Verification items for the finished model (mm, model axes). A direction names the side the tool comes from. Coordinates: 2 decimals unless noted, no trailing zeros. Order: outer loops, then holes, each group sorted by start corner. A loop starts at its lowest first (then second) coordinate and runs counter-clockwise, first axis right, second up. Notation, with made-up numbers: (-12, -2.75) -> (17, -2.75) arc R4 ccw to (17, 4.25) -> close; hole circle Ø6 at (6, 60.25). An arc over 180 degrees is marked (long way). Write each question's results on one line, items separated by ' | '. Start each with the question number.
(1) Cross-section at C-C on y = 9.5. Enter the section's corners in (x, z), and give its area (3 significant figures).
(2) Cross-section at A-A on x = 0. Give the number of separate pieces and of enclosed holes in the cut face, and give its area (3 significant figures).
(3) Cross-section at B-B on z = 15.25. Enter the section's corners in (x, y).
(4) Go/stop test with flat-tipped pins: pin 1 (2.5 mm diameter, centred on y = -6, z = 5, fed in from +X); pin 2 (1.5 mm diameter, centred on y = 0.5, z = 15, fed in from +X); pin 3 (4 mm diameter, centred on y = -6.5, z = 15, fed in from -X). Record where each tip stops, or that it passes through.
(5) Draft check along Y on faces 1 (the flat face through (0, 7.312, 9)), 2 (the cylindrical face through (-7.289, 4.196, 4.056)), 3 (the cylindrical face through (-7.289, -8.196, 10.712)). Enter one of: +Y half, -Y half, draft (parallel to the pull), parting line (faces both ways), or undercut.
(6) Set-up check for faces 4 (the flat face through (-3.95, 5, 16)), 5 (the cylindrical face through (-3.649, -9.715, 15.965)), 6 (the flat face through (3.127, 12.678, 9.232)), 7 (the flat face through (0, -2.124, 1)), 8 (the cylindrical face through (7.289, 4.196, 4.056)): record each of +Z, -Z, +X, -X, +Y, -Y from which the full face is reachable in a straight line by a thin tool's end or side.
(7) Cross-section at D-D on z = 4. Enter the section's corners in (x, y).
(8) Thickness scan on probe 1 along Y at (x, z) = (0, 13); probe 2 along Y at (x, z) = (0.25, 13.5); probe 3 along Z at (x, y) = (0, -2.45). Record the ranges inside material, lowest first. Write a range as [from, to].
```python
from build123d import *

# Parameters (mm, degrees)
F0_W         = 18
F0_H         = 16
F0_W_2       = 7.2
F0_H_2       = 3.15
F1_DEPTH     = 8
F2_R         = 6
F4_R         = 2.1
F5_DEPTH     = 10
F7_R         = 2.15
F8_DEPTH     = 5.5
F9_DEPTH     = 2.5
F10_T1_DEPTH = 35.4995000042
F12_R        = 2.15
F13_DEPTH    = 5
F14_T1_DEPTH = 7.5071501803


# Not quite as in the source:
# - a fillet or chamfer that OpenCascade refuses, or shapes differently, is made with other operations: its cross-section is extruded or revolved along the edge and cut away or added


with BuildPart() as f1:
    # F0 (on Top) → F1 (new body)
    with BuildSketch(Plane.XY):
        with Locations((0, -2)):
            Rectangle(F0_W, F0_H)
        with Locations((0, -5.225)):
            Rectangle(F0_W_2, F0_H_2, mode=Mode.SUBTRACT)
        with BuildLine():
            ThreePointArc((-1.5, -2.1236760582), (-1.1958260743, 2.3086792761), (2.6, 0))
            ThreePointArc((2.6, 0), (2.3086792761, -1.1958260743), (1.5, -2.1236760582))
            ThreePointArc((1.5, -2.1236760582), (0, -2.6), (-1.5, -2.1236760582))
        make_face(mode=Mode.SUBTRACT)
        with BuildLine():
            Line((1.5, -2.1236760582), (-1.5, -2.1236760582))
            ThreePointArc((-1.5, -2.1236760582), (0, -2.6), (1.5, -2.1236760582))
        make_face()
    extrude(amount=F1_DEPTH)

    # F2
    f2_edges = [f1.edges().sort_by_distance(p)[0] for p in [
        (9, -10, 4),
        (-9, -10, 4),
        (9, 6, 4),
        (-9, 6, 4),
    ]]
    fillet(f2_edges, radius=F2_R)

    # F4 (on offset) → F5 (cut)
    with BuildSketch(Plane.XZ.offset(10)):
        with Locations((0, 4)):
            Circle(F4_R)
    extrude(amount=-F5_DEPTH, mode=Mode.SUBTRACT)

    # F7 (on offset) → F8 (join)
    with BuildSketch(Plane.XY.offset(8)):
        Polygon((-9, 20), (-9, 0), (-9, -4), (-9, -10), (-3, -10), (3, -10), (9, -10), (9, -4), (9, 0), (9, 20), align=None)
        with BuildLine():
            ThreePointArc((-1.5, -2.1236760582), (0, 2.6), (1.5, -2.1236760582))
            Line((1.5, -2.1236760582), (-1.5, -2.1236760582))
        make_face(mode=Mode.SUBTRACT)
        with BuildLine():
            ThreePointArc((2.075, 14.5), (3.5940054257, 12.9809945743), (4.15, 10.9059945743))
            ThreePointArc((4.15, 10.9059945743), (3.5940054257, 8.8309945743), (2.075, 7.3119891486))
            ThreePointArc((2.075, 7.3119891486), (0, 6.7559945743), (-2.075, 7.3119891486))
            ThreePointArc((-2.075, 7.3119891486), (-3.5940054257, 8.8309945743), (-4.15, 10.9059945743))
            ThreePointArc((-4.15, 10.9059945743), (-3.5940054257, 12.9809945743), (-2.075, 14.5))
            ThreePointArc((-2.075, 14.5), (0, 15.0559945743), (2.075, 14.5))
        make_face(mode=Mode.SUBTRACT)
        with BuildLine():
            ThreePointArc((-4.15, 10.9059945743), (-3.5940054257, 8.8309945743), (-2.075, 7.3119891486))
            Line((-2.075, 7.3119891486), (-4.15, 10.9059945743))
        make_face()
        with BuildLine():
            Line((-4.15, 10.9059945743), (-2.075, 14.5))
            ThreePointArc((-2.075, 14.5), (-3.5940054257, 12.9809945743), (-4.15, 10.9059945743))
        make_face()
        with BuildLine():
            Line((-2.075, 14.5), (2.075, 14.5))
            ThreePointArc((2.075, 14.5), (0, 15.0559945743), (-2.075, 14.5))
        make_face()
        with BuildLine():
            Line((2.075, 14.5), (4.15, 10.9059945743))
            ThreePointArc((4.15, 10.9059945743), (3.5940054257, 12.9809945743), (2.075, 14.5))
        make_face()
        with BuildLine():
            ThreePointArc((2.075, 7.3119891486), (3.5940054257, 8.8309945743), (4.15, 10.9059945743))
            Line((4.15, 10.9059945743), (2.075, 7.3119891486))
        make_face()
        with BuildLine():
            ThreePointArc((-2.075, 7.3119891486), (0, 6.7559945743), (2.075, 7.3119891486))
            Line((2.075, 7.3119891486), (-2.075, 7.3119891486))
        make_face()
        Polygon((2.075, 7.3119891486), (4.15, 10.9059945743), (2.075, 14.5), (-2.075, 14.5), (-4.15, 10.9059945743), (-2.075, 7.3119891486), align=None)
        with Locations((0, 10.9059945743)):
            Circle(F7_R, mode=Mode.SUBTRACT)
    extrude(amount=F8_DEPTH)

    # F7 (on offset) → F9 (cut)
    with BuildSketch(Plane.XY.offset(8)):
        Polygon((2.075, 7.3119891486), (4.15, 10.9059945743), (2.075, 14.5), (-2.075, 14.5), (-4.15, 10.9059945743), (-2.075, 7.3119891486), align=None)
        with Locations((0, 10.9059945743)):
            Circle(F7_R, mode=Mode.SUBTRACT)
    extrude(amount=F9_DEPTH, mode=Mode.SUBTRACT)

    # F10: fillet of radius 6 on 4 edges, made by hand

    # F10_s2 → F10_t1 (cut)
    with BuildSketch(Plane.XY.offset(-6.9997500021)):
        with BuildLine():
            ThreePointArc((-9.0001, -4.0001), (-7.2427406871, -8.2427406871), (-3.0001, -10.0001))
            Line((-3.0001, -10.0001), (-3.0001, -10.1201))
            ThreePointArc((-3.0001, -10.1201), (-6.00005, -10.12), (-9, -10.12))
            Line((-9, -10.12), (-9.12, -10))
            ThreePointArc((-9.12, -10), (-9.12, -7.00005), (-9.1201, -4.0001))
            Line((-9.1201, -4.0001), (-9.0001, -4.0001))
        make_face()
        with BuildLine():
            ThreePointArc((9.0001, -4.0001), (7.2427406871, -8.2427406871), (3.0001, -10.0001))
            Line((3.0001, -10.0001), (3.0001, -10.1201))
            ThreePointArc((3.0001, -10.1201), (6.00005, -10.12), (9, -10.12))
            Line((9, -10.12), (9.12, -10))
            ThreePointArc((9.12, -10), (9.12, -7.00005), (9.1201, -4.0001))
            Line((9.1201, -4.0001), (9.0001, -4.0001))
        make_face()
        with BuildLine():
            ThreePointArc((9.0001, 14.0001), (7.2427406871, 18.2427406871), (3.0001, 20.0001))
            Line((3.0001, 20.0001), (3.0001, 20.1201))
            ThreePointArc((3.0001, 20.1201), (6.00005, 20.12), (9, 20.12))
            Line((9, 20.12), (9.12, 20))
            ThreePointArc((9.12, 20), (9.12, 17.00005), (9.1201, 14.0001))
            Line((9.1201, 14.0001), (9.0001, 14.0001))
        make_face()
        with BuildLine():
            ThreePointArc((-9.0001, 14.0001), (-7.2427406871, 18.2427406871), (-3.0001, 20.0001))
            Line((-3.0001, 20.0001), (-3.0001, 20.1201))
            ThreePointArc((-3.0001, 20.1201), (-6.00005, 20.12), (-9, 20.12))
            Line((-9, 20.12), (-9.12, 20))
            ThreePointArc((-9.12, 20), (-9.12, 17.00005), (-9.1201, 14.0001))
            Line((-9.1201, 14.0001), (-9.0001, 14.0001))
        make_face()
    extrude(amount=F10_T1_DEPTH, mode=Mode.SUBTRACT)

    # F12 (on offset) → F13 (join)
    with BuildSketch(Plane.XY.offset(13.5)):
        with BuildLine():
            Line((-3.95, 19.9243143063), (-3.95, -9.9243143063))
            ThreePointArc((-3.95, -9.9243143063), (-3.4765050693, -9.9810486471), (-3, -10))
            Line((-3, -10), (3, -10))
            ThreePointArc((3, -10), (3.4765050693, -9.9810486471), (3.95, -9.9243143063))
            Line((3.95, -9.9243143063), (3.95, 19.9243143063))
            ThreePointArc((3.95, 19.9243143063), (3.4765050693, 19.9810486471), (3, 20))
            Line((3, 20), (-3, 20))
            ThreePointArc((-3, 20), (-3.4765050693, 19.9810486471), (-3.95, 19.9243143063))
        make_face()
        with BuildLine():
            Line((1.5, -2.1236760582), (-1.5, -2.1236760582))
            ThreePointArc((-1.5, -2.1236760582), (0, 2.6), (1.5, -2.1236760582))
        make_face(mode=Mode.SUBTRACT)
        with Locations((0, 10.9059945743)):
            Circle(F12_R, mode=Mode.SUBTRACT)
    extrude(amount=F13_DEPTH)

    # F14: fillet of radius 1 on 4 edges, made by hand

    # F14_s2 → F14_t1 (cut)
    with BuildSketch(Plane.XY.offset(13.5)):
        with BuildLine():
            ThreePointArc((3.95, -9), (3.6571067812, -9.7071067812), (2.95, -10))
            Line((2.95, -10), (2.95, -10.1))
            ThreePointArc((2.95, -10.1), (3, -10.1), (3.9658333333, -10.0230528781))
            Line((3.9658333333, -10.0230528781), (4.05, -9.9243143063))
            Line((4.05, -9.9243143063), (4.05, -9))
            Line((4.05, -9), (3.95, -9))
        make_face()
        with BuildLine():
            ThreePointArc((-2.95, -10), (-3.6571067812, -9.7071067812), (-3.95, -9))
            Line((-3.95, -9), (-4.05, -9))
            Line((-4.05, -9), (-4.05, -9.9243143063))
            Line((-4.05, -9.9243143063), (-3.9658333333, -10.0230528781))
            ThreePointArc((-3.9658333333, -10.0230528781), (-3, -10.1), (-2.95, -10.1))
            Line((-2.95, -10.1), (-2.95, -10))
        make_face()
        with BuildLine():
            ThreePointArc((2.95, 20), (3.6571067812, 19.7071067812), (3.95, 19))
            Line((3.95, 19), (4.05, 19))
            Line((4.05, 19), (4.05, 19.9243143063))
            Line((4.05, 19.9243143063), (3.9658333333, 20.0230528781))
            ThreePointArc((3.9658333333, 20.0230528781), (3, 20.1), (2.95, 20.1))
            Line((2.95, 20.1), (2.95, 20))
        make_face()
        with BuildLine():
            ThreePointArc((-2.95, 20), (-3.6571067812, 19.7071067812), (-3.95, 19))
            Line((-3.95, 19), (-4.05, 19))
            Line((-4.05, 19), (-4.05, 19.9243143063))
            Line((-4.05, 19.9243143063), (-3.9658333333, 20.0230528781))
            ThreePointArc((-3.9658333333, 20.0230528781), (-3, 20.1), (-2.95, 20.1))
            Line((-2.95, 20.1), (-2.95, 20))
        make_face()
    extrude(amount=F14_T1_DEPTH, mode=Mode.SUBTRACT)


solid = f1.part
```
Results are:
1) outline: (-9, 8) -> (-3.34, 8) -> (-3.34, 10.5) -> (-1.63, 10.5) -> (-1.63, 18.5) -> (-3.95, 18.5) -> (-3.95, 13.5) -> (-9, 13.5) -> close; (1.63, 10.5) -> (3.34, 10.5) -> (3.34, 8) -> (9, 8) -> (9, 13.5) -> (3.95, 13.5) -> (3.95, 18.5) -> (1.63, 18.5) -> close | area: 95.8 mm2
2) separate pieces: 5 | enclosed holes: 0 | area: 258 mm2
3) outline: (-3.95, -9) arc R1 ccw to (-2.95, -10) -> (2.95, -10) arc R1 ccw to (3.95, -9) -> (3.95, 19) arc R1 ccw to (2.95, 20) -> (-2.95, 20) arc R1 ccw to (-3.95, 19) -> close; hole circle Ø4.3 at (0, 10.91); hole (-1.5, -2.12) -> (1.5, -2.12) arc R2.6 ccw (long way) to start
4) pin 1: stops at x = 8.95 | pin 2: stops at x = 3.95 | pin 3: stops at x = -8.88
5) face 1: undercut | face 2: +Y half | face 3: -Y half
6) face 4: +Z, -X, +Y, -Y | face 5: +Z, -X, -Y | face 6: -Z | face 7: +Z, -Z | face 8: -Z, +X, +Y
7) outline: (-9, -4) arc R6 ccw to (-3, -10) -> (-2.1, -10) -> (-2.1, -6.8) -> (-3.6, -6.8) -> (-3.6, -3.65) -> (-2.1, -3.65) -> (-2.1, -1.53) arc R2.6 cw (long way) to (2.1, -1.53) -> (2.1, -3.65) -> (3.6, -3.65) -> (3.6, -6.8) -> (2.1, -6.8) -> (2.1, -10) -> (3, -10) arc R6 ccw to (9, -4) -> (9, 0) arc R6 ccw to (3, 6) -> (-3, 6) arc R6 ccw to (-9, 0) -> close
8) probe 1: y = [-10, -2.12], [2.6, 8.76], [13.06, 20] | probe 2: y = [-10, -2.12], [2.59, 8.77], [13.04, 20] | probe 3: z = [0, 1.9], [6.1, 18.5]
